from build123d import *

# Parameters (mm, degrees)
BOSS_EXTRUDE1_DEPTH      = 25.4
SKETCH3_R                = 1.625000052
CUT_EXTRUDE1_HOLES_DEPTH = 39.978915227


with BuildPart() as part:
    # Sketch2 → Boss-Extrude1 (new body)
    with BuildSketch(Plane.XY):
        with BuildLine():
            Line((-26.67, 0), (-17.8435, 0))
            ThreePointArc((-17.8435, 0), (-17.657932489, 2.566692903), (-17.105089659, 5.08))
            Line((-17.105089659, 5.08), (-17.8435, 5.08))
            Line((-17.8435, 5.08), (-26.67, 5.08))
            Line((-26.67, 5.08), (-26.67, 0))
        make_face()
        with BuildLine():
            Line((-17.8435, 0), (-12.7635, 0))
            ThreePointArc((-12.7635, 0), (-12.497093116, 2.594146471), (-11.708993648, 5.08))
            Line((-11.708993648, 5.08), (-17.105089659, 5.08))
            ThreePointArc((-17.105089659, 5.08), (-17.657932489, 2.566692903), (-17.8435, 0))
        make_face()
        with BuildLine():
            Line((-17.105089659, 5.08), (-11.708993648, 5.08))
            ThreePointArc((-11.708993648, 5.08), (0, 12.7635), (11.708993648, 5.08))
            Line((11.708993648, 5.08), (17.105089659, 5.08))
            ThreePointArc((17.105089659, 5.08), (0, 17.8435), (-17.105089659, 5.08))
        make_face()
        with BuildLine():
            ThreePointArc((11.708993648, 5.08), (12.497093116, 2.594146471), (12.7635, 0))
            Line((12.7635, 0), (17.8435, 0))
            ThreePointArc((17.8435, 0), (17.657932489, 2.566692903), (17.105089659, 5.08))
            Line((17.105089659, 5.08), (11.708993648, 5.08))
        make_face()
        with BuildLine():
            ThreePointArc((17.105089659, 5.08), (17.657932489, 2.566692903), (17.8435, 0))
            Line((17.8435, 0), (26.67, 0))
            Line((26.67, 0), (26.67, 5.08))
            Line((26.67, 5.08), (17.8435, 5.08))
            Line((17.8435, 5.08), (17.105089659, 5.08))
        make_face()
    extrude(amount=BOSS_EXTRUDE1_DEPTH)

    # Sketch3 → Cut-Extrude1 Holes (cut, through all)
    with BuildSketch(Plane(origin=(0, 5.08, 0), x_dir=(1, 0, 0), z_dir=(0, 1, 0))):
        with Locations((-22.86, -6.99999997)):
            Circle(SKETCH3_R)
        with BuildLine():
            Line((-22.86, -5.0162412), (-23.792061739, -5.668877855))
            ThreePointArc((-23.792061739, -5.668877855), (-22.86, -5.374999918), (-21.927938261, -5.668877855))
            Line((-21.927938261, -5.668877855), (-22.86, -5.0162412))
        make_face()
        with Locations((-22.86, -18.999999846)):
            Circle(SKETCH3_R)
        with BuildLine():
            Line((-21.927938261, -17.668877731), (-22.86, -17.016241076))
            Line((-22.86, -17.016241076), (-23.792061739, -17.668877731))
            ThreePointArc((-23.792061739, -17.668877731), (-22.86, -17.374999794), (-21.927938261, -17.668877731))
        make_face()
        with Locations((22.86, -18.999999846)):
            Circle(SKETCH3_R)
        with BuildLine():
            Line((23.792061739, -17.668877731), (22.86, -17.016241076))
            Line((22.86, -17.016241076), (21.927938261, -17.668877731))
            ThreePointArc((21.927938261, -17.668877731), (22.86, -17.374999794), (23.792061739, -17.668877731))
        make_face()
        with Locations((22.86, -6.99999997)):
            Circle(SKETCH3_R)
        with BuildLine():
            Line((23.792061739, -5.668877855), (22.86, -5.0162412))
            Line((22.86, -5.0162412), (21.927938261, -5.668877855))
            ThreePointArc((21.927938261, -5.668877855), (22.86, -5.374999918), (23.792061739, -5.668877855))
        make_face()
    extrude(amount=-CUT_EXTRUDE1_HOLES_DEPTH, mode=Mode.SUBTRACT)


solid = part.part
Geometry check sheet. Reference: the model listing, model coordinates, mm. A direction names the side the tool comes from. Give positions to 0.01 mm unless a question says otherwise; leave off trailing zeros. Loops run counter-clockwise (first coordinate to the right, second up) from the corner with the lowest first, then second, coordinate; pieces in that order, holes last. Notation, with made-up numbers: (54, 58) -> (113, 58) arc R21 cw to (113, 83) -> close; hole circle Ø6 at (-31, 16). An arc over 180 degrees is marked (long way). Answer in a Markdown table with one row per item. Add a question column.
1) Draft check along Z on faces 1 (the face through (-23.32, 2.58, 17.34)), 2 (the face through (26.67, 3, 13)), 3 (the face through (2, 13, 0)). Enter one of: pulls with the +Z half, pulls with the -Z half, needs draft (parallel to the pull), parting line crosses it, or undercut.
2) Set-up check for faces 4 (the face through (22, 5.08, 13)), 5 (the face through (-22, 5.08, 13)), 6 (the face through (-23.32, 2.58, 5.34)): record each of +Z, -Z, +X, -X, +Y, -Y from which the full face is reachable in a straight line by a thin tool's end or side.
3) Gauge pin test, flat ends, axial feed: P1, Ø12, axis at x = 1, z = 17.5, coming from the -Y side; P2, Ø5, axis at y = 14.5, z = 20.5, coming from the -X side; P3, Ø10, axis at x = 15.5, y = 15.5, coming from the +Z side; P4, Ø1.5, axis at y = 11, z = 10.5, coming from the +X side. Record the tip position at first contact, or that the pin passes through.
4) Cross-section at B-B on y = 11.25. Record the boundary of the cut face in (x, z), and give its area (3 significant figures).
5) Cross-section at D-D on y = 5.75. Record the boundary of the cut face in (x, z), and give its area (3 significant figures).
6) Material ranges on probe 1 along Z at (x, y) = (22.86, 3.7) (3 decimals); probe 2 along X at (y, z) = (3.7, 19) (3 decimals); probe 3 along X at (y, z) = (3.35, 7) (3 decimals), recorded low to high. Write a range as from..to.
7) Cross-section at C-C on z = 4. Record the boundary of the cut face in (x, y), and give its area (3 significant figures).
8) Cross-section at A-A on z = 7. Record the boundary of the cut face in (x, y) (1 decimal), and give its area (3 significant figures).
Outcome:
| question | item | result |
|---|---|---|
| 1 | face 1 | undercut |
| 1 | face 2 | needs draft |
| 1 | face 3 | pulls with the -Z half |
| 2 | face 4 | +Z, -Z, +X, +Y |
| 2 | face 5 | +Z, -Z, -X, +Y |
| 2 | face 6 | +Y, -Y |
| 3 | P1 | stops at y = 10.67 |
| 3 | P2 | stops at x = -13.21 |
| 3 | P3 | stops at z = 25.4 |
| 3 | P4 | stops at x = 14.61 |
| 4 | outline | (-13.85, 0) -> (-6.03, 0) -> (-6.03, 25.4) -> (-13.85, 25.4) -> close; (6.03, 0) -> (13.85, 0) -> (13.85, 25.4) -> (6.03, 25.4) -> close |
| 4 | area | 397 mm^2 |
| 5 | outline | (-16.89, 0) -> (-11.39, 0) -> (-11.39, 25.4) -> (-16.89, 25.4) -> close; (11.39, 0) -> (16.89, 0) -> (16.89, 25.4) -> (11.39, 25.4) -> close |
| 5 | area | 279 mm^2 |
| 6 | probe 1 | z = 0..5.016, 8.625..17.016, 20.625..25.4 |
| 6 | probe 2 | x = -26.67..-24.485, -21.235..-12.215, 12.215..21.235, 24.485..26.67 |
| 6 | probe 3 | x = -26.67..-24.485, -21.235..-12.316, 12.316..21.235, 24.485..26.67 |
| 7 | outline | (-26.67, 0) -> (-12.76, 0) arc R12.76 cw to (12.76, 0) -> (26.67, 0) -> (26.67, 5.08) -> (17.11, 5.08) arc R17.84 ccw to (-17.11, 5.08) -> (-26.67, 5.08) -> close |
| 7 | area | 336 mm^2 |
| 8 | outline | (-26.7, 0) -> (-24.5, 0) -> (-24.5, 5.1) -> (-26.7, 5.1) -> close; (-21.2, 0) -> (-12.8, 0) arc R12.8 cw to (12.8, 0) -> (21.2, 0) -> (21.2, 5.1) -> (17.1, 5.1) arc R17.8 ccw to (-17.1, 5.1) -> (-21.2, 5.1) -> close; (24.5, 0) -> (26.7, 0) -> (26.7, 5.1) -> (24.5, 5.1) -> close |
| 8 | area | 303 mm^2 |
